The listing builds one solid part. Answer for the finished solid, in the listing's coordinates (mm). A direction names the side the tool comes from. Round coordinates to 2 decimals unless told otherwise and drop trailing zeros. Write each loop counter-clockwise with the first axis right and the second up, starting at its lowest first coordinate (ties: lowest second). Pieces come first, ordered by that corner, then holes.
Item 1: Find section A-A on y = 0. Give the vertices of the cut face in (x, z).
Item 2: Find the intervals of material crossed by probe 1 along Y at (x, z) = (17.5, 0.65); probe 2 along Z at (x, y) = (16, 1.5); probe 3 along Z at (x, y) = (4, -1), in increasing order.
Item 3: Each of these flat-tipped pins is pushed along its axis until it touches: pin 1 (0.8 mm diameter, centred on x = -15, z = 0.5, fed in from +Y); pin 2 (1 mm diameter, centred on x = -10.5, z = 1, fed in from -Y); pin 3 (0.5 mm diameter, centred on x = 2, y = 8, fed in from -Z); pin 4 (5.5 mm diameter, centred on x = 1.5, y = -14, fed in from +Z). Where does it stop, or does it pass through?
Item 4: Find section D-D on z = 5.5. Give the vertices of the cut face in (x, y).
Item 5: Find section B-B on x = 0. Give the vertices of the cut face in (y, z).
Item 6: Find section C-C on x = 18. Give the vertices of the cut face in (y, z), then the cut area to 3 significant figures.
Item 7: For a pull along X with two mould halves and no side action, classify faces 1 (the face through (0, 8, -10)), 2 (the face through (-19.1, -1.2, 0.5)), 3 (the face through (6.36, 12.47, 9.37)), 4 (the face through (-1.5, 8, -7)) as +X half, -X half, draft (parallel to the pull), parting line (faces both ways), or undercut.
Item 8: A tool of negligible diameter and unlimited length cuts with its end or side. For faces 5 (the face through (1.5, 8, -7)), 6 (the face through (15.5, -3.5, 0.5)), 7 (the face through (15.6, 3.5, 0.5)), 8 (the face through (-0.59, 12.46, -0.74)), from which of +Z, -Z, +X, -X, +Y, -Y can it reach the whole face along a straight path? Write none if from no direction.
```python
from build123d import *

# Parameters (mm, degrees)
ESQUISSE1_R             = 2
BOSS_EXTRU_1_DEPTH      = 1
ESQUISSE1_3_R           = 14
ESQUISSE1_3_R_2         = 4.5
ESQUISSE1_3_R_3         = 2.5
ESQUISSE1_3_R_4         = 1.5
BOSS_EXTRU_2_DEPTH      = 19
BOSS_EXTRU_3_DEPTH      = 16
ESQUISSE1_5_R           = 4.5
BOSS_EXTRU_4_DEPTH      = 1.5
ESQUISSE1_6_R           = 2.5
BOSS_EXTRU_5_DEPTH      = 10
ESQUISSE2_W             = 1
ESQUISSE2_H             = 5
ENL_V_MAT_EXTRU_1_DEPTH = 6


with BuildPart() as part:
    # Esquisse1 → Boss.-Extru.1 (new body)
    with BuildSketch(Plane.XY):
        with BuildLine():
            Line((-7.3, -11.94612908), (-7.3, -17))
            Line((-7.3, -17), (7.3, -17))
            Line((7.3, -17), (7.3, -11.94612908))
            ThreePointArc((7.3, -11.94612908), (11.250406053, -8.332368429), (13.555441712, -3.5))
            Line((13.555441712, -3.5), (17.5, -3.5))
            ThreePointArc((17.5, -3.5), (21, 0), (17.5, 3.5))
            Line((17.5, 3.5), (13.555441712, 3.5))
            ThreePointArc((13.555441712, 3.5), (0, 14), (-13.555441712, 3.5))
            Line((-13.555441712, 3.5), (-17.5, 3.5))
            ThreePointArc((-17.5, 3.5), (-21, 0), (-17.5, -3.5))
            Line((-17.5, -3.5), (-13.555441712, -3.5))
            ThreePointArc((-13.555441712, -3.5), (-11.250406053, -8.332368429), (-7.3, -11.94612908))
        make_face()
        with Locations((-17.5, 0)):
            Circle(ESQUISSE1_R, mode=Mode.SUBTRACT)
        with Locations((17.5, 0)):
            Circle(ESQUISSE1_R, mode=Mode.SUBTRACT)
    extrude(amount=BOSS_EXTRU_1_DEPTH)

    # Esquisse1_3 → Boss.-Extru.2 (add)
    # profile 1 of 4: a face of its own
    with BuildSketch(Plane.XY):
        with Locations(Location((0, 0, 0), (0, 0, 165.522487814))):
            Circle(ESQUISSE1_3_R)
        with Locations((0, 8)):
            Circle(ESQUISSE1_3_R_2, mode=Mode.SUBTRACT)
    # profile 2 of 4: a face of its own
    with BuildSketch(Plane.XY):
        with Locations((0, 8)):
            Circle(ESQUISSE1_3_R_2)
        with Locations((0, 8)):
            Circle(ESQUISSE1_3_R_3, mode=Mode.SUBTRACT)
    # profile 3 of 4: a face of its own
    with BuildSketch(Plane.XY):
        with Locations((0, 8)):
            Circle(ESQUISSE1_3_R_3)
        with Locations((0, 8)):
            Circle(ESQUISSE1_3_R_4, mode=Mode.SUBTRACT)
    # profile 4 of 4: a face of its own
    with BuildSketch(Plane.XY):
        with Locations((0, 8)):
            Circle(ESQUISSE1_3_R_4)
    extrude(amount=BOSS_EXTRU_2_DEPTH)

    # Esquisse1_4 → Boss.-Extru.3 (add)
    with BuildSketch(Plane.XY):
        with BuildLine():
            Line((-7.3, -11.94612908), (-7.3, -17))
            Line((-7.3, -17), (7.3, -17))
            Line((7.3, -17), (7.3, -11.94612908))
            ThreePointArc((7.3, -11.94612908), (0, -14), (-7.3, -11.94612908))
        make_face()
    extrude(amount=BOSS_EXTRU_3_DEPTH)

    # Esquisse1_5 → Boss.-Extru.4 (add)
    with BuildSketch(Plane.XY):
        with Locations((0, 8)):
            Circle(ESQUISSE1_5_R)
    extrude(amount=-BOSS_EXTRU_4_DEPTH)

    # Esquisse1_6 → Boss.-Extru.5 (add)
    with BuildSketch(Plane.XY):
        with Locations((0, 8)):
            Circle(ESQUISSE1_6_R)
    extrude(amount=-BOSS_EXTRU_5_DEPTH)

    # Esquisse2 → Enl_v. mat.-Extru.1 (cut)
    with BuildSketch(Plane(origin=(0, 0, -10), x_dir=(-1, 0, 0), z_dir=(0, 0, -1))):
        with Locations((2, 8)):
            Rectangle(ESQUISSE2_W, ESQUISSE2_H)
        with Locations((-2, 8)):
            Rectangle(ESQUISSE2_W, ESQUISSE2_H)
    extrude(amount=-ENL_V_MAT_EXTRU_1_DEPTH, mode=Mode.SUBTRACT)


solid = part.part
```
Check values:
1. outline: (-21, 0) - (-19.5, 0) - (-19.5, 1) - (-21, 1) - close; (-15.5, 0) - (15.5, 0) - (15.5, 1) - (14, 1) - (14, 19) - (-14, 19) - (-14, 1) - (-15.5, 1) - close; (19.5, 0) - (21, 0) - (21, 1) - (19.5, 1) - close
2. probe 1: y = -3.5 to -2, 2 to 3.5
2. probe 2: z = 0 to 1
2. probe 3: z = 0 to 19
3. pin 1: stops at y = 3.5
3. pin 2: stops at y = -9.8
3. pin 3: stops at z = -4
3. pin 4: stops at z = 19
4. outline: (-7.3, -17) - (7.3, -17) - (7.3, -11.95) arc R14 ccw (long way) to (-7.3, -11.95) - close
5. outline: (-17, 0) - (3.5, 0) - (3.5, -1.5) - (5.5, -1.5) - (5.5, -10) - (10.5, -10) - (10.5, -1.5) - (12.5, -1.5) - (12.5, 0) - (14, 0) - (14, 19) - (-14, 19) - (-14, 16) - (-17, 16) - close
6. outline: (-3.46, 0) - (-1.94, 0) - (-1.94, 1) - (-3.46, 1) - close; (1.94, 0) - (3.46, 0) - (3.46, 1) - (1.94, 1) - close
6. area: 3.06 mm2
7. face 1: draft
7. face 2: undercut
7. face 3: parting line
7. face 4: -X half
8. face 5: -Z, +X, +Y, -Y
8. face 6: +Z, -Z, +X, -Y
8. face 7: +Z, -Z, +X, +Y
8. face 8: -Z
